Could you check a few things on this model? Use its own coordinates, in mm. Face numbers are marked on the shaded views. A direction names the side the tool comes from. Coordinates: 2 decimals unless noted, no trailing zeros. Order: outer loops, then holes, each group sorted by start corner. A loop starts at its lowest first (then second) coordinate and runs counter-clockwise, first axis right, second up. Notation, with made-up numbers: (43, 47) -> (56, 47) arc R16 ccw to (56, 72) -> close; hole circle Ø9 at (79.25, 62). An arc over 180 degrees is marked (long way). Use a Markdown table: item, result. Add a question column.
1) If I drill on L1, parallel to X at y = 0, z = -6; L2, parallel to X at y = 12, z = 5.5; L3, parallel to X at y = 14.5, z = 25.5, over which ranges is the centre line in solid material (lowest first)? Write a range as [from, to].
2) Which directions (+Z, -Z, +X, -X, +Y, -Y) give clear straight access to the entire face, cutting with the end or side of a thin tool? Please do the marked faces 1, 2 and 3.
3) If we section it at D-D (x = 155): Write out the boundary of the cut face in (y, z).
4) If we section it at B-B (z = 0): Write out the boundary of the cut face in (x, y).
5) If we section it at C-C (x = 83): Write out the boundary of the cut face in (y, z).
6) Will these pins go through, and if not, where does the flat tip stop? pin 1 Ø6 at (x, z) = (52.5, 10.5) entering from +Y; pin 2 Ø10 at (x, z) = (116.5, 18.5) entering from +Y; pin 3 Ø6 at (x, y) = (58, 7) entering from +Z; pin 4 Ø1 at (y, z) = (2.5, 5.5) entering from -X.
7) If we section it at A-A (y = 0): Write out the boundary of the cut face in (x, z), plus the area to 4 significant figures.
```python
from build123d import *

# Parameters (mm, degrees)
SKETCH_2_R          = 5
CUT_EXTRUDE_1_DEPTH = 209.32666656


with BuildPart() as part:
    # 草图1 → 旋转1 (revolve)
    with BuildSketch(Plane.XY, mode=Mode.PRIVATE) as revolve_1_sk:
        Polygon((0, 0), (200, 0), (200, 15), (165, 20), (60, 20), (60, 30), (50, 30), (50, 10), (0, 10), align=None)
    revolve(revolve_1_sk.sketch.rotate(Axis((0, 0, 0), (1, 0, 0)), 90), axis=Axis((0, 0, 0), (1, 0, 0)))

    # 草图2 → 切除-拉伸1 (cut, through all)
    with BuildSketch(Plane.XY.offset(20)):
        with Locations((155, 0)):
            Circle(SKETCH_2_R)
    extrude(amount=-CUT_EXTRUDE_1_DEPTH, mode=Mode.SUBTRACT)


solid = part.part
```
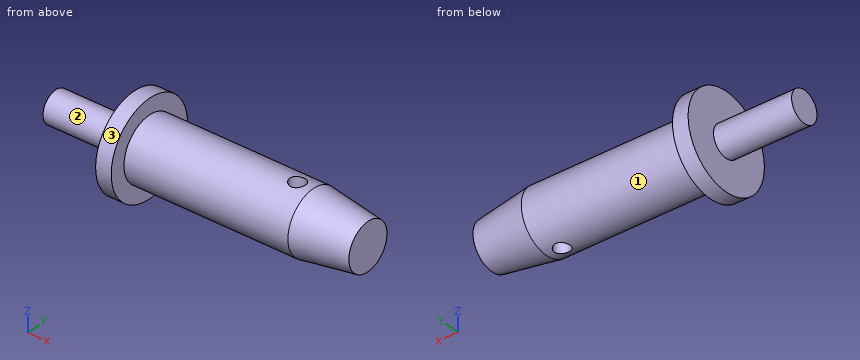
Answer sheet:
| question | item | result |
|---|---|---|
| 1 | L1 | [0, 150], [160, 200] |
| 1 | L2 | [50, 200] |
| 1 | L3 | [50, 60] |
| 2 | face 1 | +X |
| 2 | face 2 | -X |
| 2 | face 3 | +X, -X |
| 3 | outline | (-5, -19.36) -> (-5, 19.36) arc R20 ccw to start; (5, -19.36) arc R20 ccw to (5, 19.36) -> close |
| 4 | outline | (0, -10) -> (50, -10) -> (50, -30) -> (60, -30) -> (60, -20) -> (165, -20) -> (200, -15) -> (200, 15) -> (165, 20) -> (60, 20) -> (60, 30) -> (50, 30) -> (50, 10) -> (0, 10) -> close; hole circle Ø10 at (155, 0) |
| 5 | outline | circle Ø40 at (0, 0) |
| 6 | pin 1 | y = 29.05 |
| 6 | pin 2 | y = 14.76 |
| 6 | pin 3 | z = 29.73 |
| 6 | pin 4 | x = 0 |
| 7 | outline | (0, -10) -> (50, -10) -> (50, -30) -> (60, -30) -> (60, -20) -> (150, -20) -> (150, 20) -> (60, 20) -> (60, 30) -> (50, 30) -> (50, 10) -> (0, 10) -> close; (160, -20) -> (165, -20) -> (200, -15) -> (200, 15) -> (165, 20) -> (160, 20) -> close |
| 7 | area | 6,625 mm2 |
